Can you work these out from the drawing? Everything is in mm from the part's minimum corner. Round coordinates to 2 decimals unless told otherwise and drop trailing zeros. Loops run counter-clockwise (first coordinate to the right, second up) from the corner with the lowest first, then second, coordinate; pieces in that order, holes last. Notation, with made-up numbers: (31.5, 73) -> (78.5, 73) arc R20 cw to (78.5, 78) -> close; hole circle Ø6 at (-13.5, 46.5). An arc over 180 degrees is marked (long way). Answer as a JSON object with one key per item and string values.
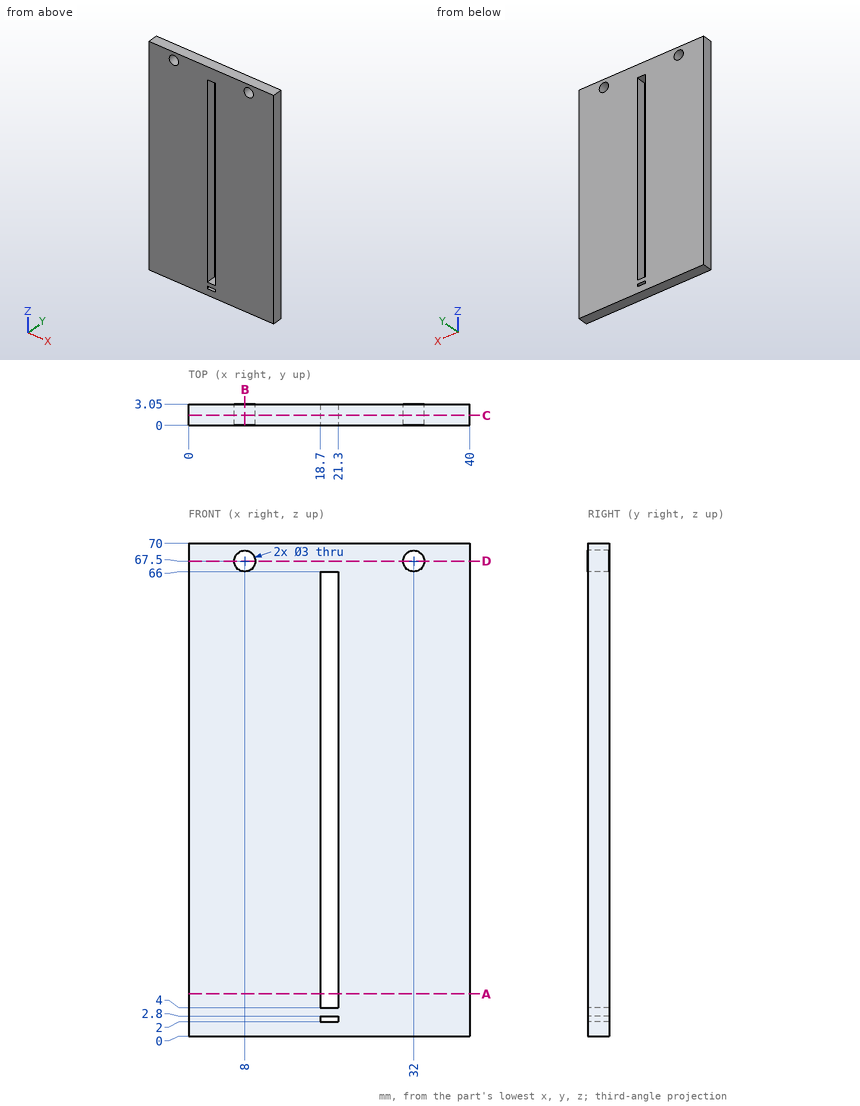
Q1. I want a section at B-B, the plane x = 8. Write out the boundary of the cut face in (y, z).
Determined:
{"outline": "(0, 0) -> (3.05, 0) -> (3.05, 66) -> (0, 66) -> close; (0, 69) -> (3.05, 69) -> (3.05, 70) -> (0, 70) -> close"}
Q2. I'm going to push a flat-ended pin straight in: pin 1 (1.8 mm diameter, centred on x = 32, z = 67.5, fed in from +Y). Where does the tip first touch, or does it pass through?
Determined:
{"pin 1": "through"}
Q3. If I drill on L1, parallel to X at y = 1.45, z = 67.5; L2, parallel to Z at x = 20, y = 0.9; L3, parallel to X at y = 2.95, z = 13.5, over which ranges is the centre line in solid material (lowest first)? Write a range as [from, to].
Determined:
{"L1": "[0, 6.5], [9.5, 30.5], [33.5, 40]", "L2": "[0, 2], [2.8, 4], [66, 70]", "L3": "[0, 18.7], [21.3, 40]"}
Q4. I want a section at D-D, the plane z = 67.5. Write out the boundary of the cut face in (x, y).
Determined:
{"outline": "(0, 0) -> (6.5, 0) -> (6.5, 3.05) -> (0, 3.05) -> close; (9.5, 0) -> (30.5, 0) -> (30.5, 3.05) -> (9.5, 3.05) -> close; (33.5, 0) -> (40, 0) -> (40, 3.05) -> (33.5, 3.05) -> close"}
Q5. I want a section at C-C, the plane y = 1.45. Write out the boundary of the cut face in (x, z), then the cut area to 3 significant figures.
Determined:
{"outline": "(0, 0) -> (40, 0) -> (40, 70) -> (0, 70) -> close; hole circle Ø3 at (8, 67.5); hole (18.7, 2) -> (21.3, 2) -> (21.3, 2.8) -> (18.7, 2.8) -> close; hole (18.7, 4) -> (21.3, 4) -> (21.3, 66) -> (18.7, 66) -> close; hole circle Ø3 at (32, 67.5)", "area": "2,620 mm²"}
Q6. I want a section at A-A, the plane z = 6. Write out the boundary of the cut face in (x, y), then the cut area to 3 significant figures.
Determined:
{"outline": "(0, 0) -> (18.7, 0) -> (18.7, 3.05) -> (0, 3.05) -> close; (21.3, 0) -> (40, 0) -> (40, 3.05) -> (21.3, 3.05) -> close", "area": "114 mm²"}
